For this review, take the finished solid that the model builds, in its own axes (mm). Round coordinates to 2 decimals unless told otherwise and drop trailing zeros. Write each loop counter-clockwise with the first axis right and the second up, starting at its lowest first coordinate (ties: lowest second). Pieces come first, ordered by that corner, then holes.
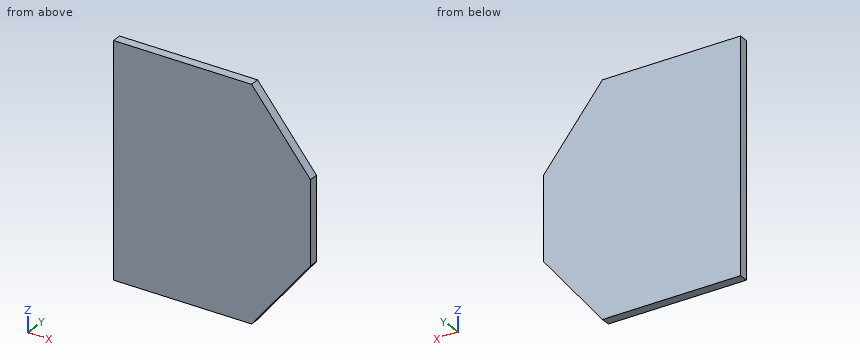
from build123d import *

# Parameters (mm, degrees)
BOSS_EXTRUDE1_DEPTH = 5
SKETCH3_W           = 36
SKETCH3_H           = 90
CUT_EXTRUDE1_DEPTH  = 10


with BuildPart() as part:
    # Sketch1 → Boss-Extrude1 (new, symmetric)
    with BuildSketch(Plane(origin=(0, 0, 0), x_dir=(1, 0, 0), z_dir=(0, 1, 0))):
        Polygon((75, 125), (175, 0), (75, -125), (-75, -125), (-75, 125), align=None)
    extrude(amount=BOSS_EXTRUDE1_DEPTH, both=True)

    # Sketch3 → Cut-Extrude1 (cut)
    with BuildSketch(Plane(origin=(0, 5, 0), x_dir=(1, 0, 0), z_dir=(0, 1, 0))):
        with Locations((157, 0)):
            Rectangle(SKETCH3_W, SKETCH3_H)
    extrude(amount=-CUT_EXTRUDE1_DEPTH, mode=Mode.SUBTRACT)


solid = part.part
(1) We need section C-C, the plane x = 82. Give the boundary of the cut face in (y, z).
Geometry check:
outline: (-5, -116.25) - (5, -116.25) - (5, 116.25) - (-5, 116.25) - close
(2) For pin 1 Ø3 at (y, z) = (-2.5, 89.5) entering from +X, flat-tipped, find the tip position at first contact; note if it passes through.
Geometry check:
pin 1: stops at x = 104.6
(3) We need section A-A, the plane y = -0.5. Give the boundary of the cut face in (x, z).
Geometry check:
outline: (-75, -125) - (75, -125) - (139, -45) - (139, 45) - (75, 125) - (-75, 125) - close
(4) For line 1 along X through (y, z) = (-0.25, 57); line 2 along Z through (x, y) = (92, 2.5); line 3 along X through (y, z) = (-1.25, 104), list the stretches that pass through material, from the lowest coordinate up.
Geometry check:
line 1: x = -75 to 129.4
line 2: z = -103.75 to 103.75
line 3: x = -75 to 91.8
(5) We need section B-B, the plane z = 88. Give the boundary of the cut face in (x, y).
Geometry check:
outline: (-75, -5) - (104.6, -5) - (104.6, 5) - (-75, 5) - close
